from build123d import *

# Parameters (mm, degrees)
CHAMFER_1_SIZE      = 0.5
SKETCH_2_R          = 1.65
CUT_EXTRUDE_1_DEPTH = 10
SKETCH_3_R          = 1.65
CUT_EXTRUDE_2_DEPTH = 10


with BuildPart() as part:
    # 草图1 → 旋转1 (revolve)
    with BuildSketch(Plane(origin=(0, 0, 0), x_dir=(1, 0, 0), z_dir=(0, 1, 0))):
        Polygon((14, 8), (0, 8), (0, 2.5), (9, 2.5), (9, 4), (14, 4), align=None)
    revolve(axis=Axis((-5, 0, 0), (1, 0, 0)))

    # 倒角1
    chamfer_1_edges = [part.edges().sort_by_distance(p)[0] for p in [
        (14, 0, 4),
        (9, 0, 2.5),
        (0, 0, 2.5),
        (0, 0, 8),
        (14, 0, 8),
    ]]
    chamfer(chamfer_1_edges, length=CHAMFER_1_SIZE)

    # 草图2 → 切除-拉伸1 (cut)
    with BuildSketch(Plane(origin=(0, 0, 0), x_dir=(1, 0, 0), z_dir=(0, 1, 0))):
        with Locations((3, 0)):
            Circle(SKETCH_2_R)
        with Locations((11, 0)):
            Circle(SKETCH_2_R)
    extrude(amount=-CUT_EXTRUDE_1_DEPTH, mode=Mode.SUBTRACT)

    # 草图3 → 切除-拉伸2 (cut)
    with BuildSketch(Plane.XY):
        with Locations((3, 0)):
            Circle(SKETCH_3_R)
        with Locations((11, 0)):
            Circle(SKETCH_3_R)
    extrude(amount=-CUT_EXTRUDE_2_DEPTH, mode=Mode.SUBTRACT)


solid = part.part
Can you work these out from the model? Positions are in its coordinate system, mm. A direction names the side the tool comes from. Round coordinates to 2 decimals unless told otherwise and drop trailing zeros. Order: outer loops, then holes, each group sorted by start corner. A loop starts at its lowest first (then second) coordinate and runs counter-clockwise, first axis right, second up. Notation, with made-up numbers: M 60.5,62.25 L 110.5,62.25 A22 ccw 110.5,91.25 Z; hole C 2.5,15.5 d5. An arc over 180 degrees is marked long. Use a Markdown table: item, result.
1) I'm going to push flat-ended pins straight in: P1, Ø2.5, axis at y = 1, z = 0.5, coming from the +X side; P2, Ø3, axis at x = 11, y = -0.5, coming from the -Z side; P3, Ø6.5, axis at y = 0, z = 0, coming from the +X side; P4, Ø4, axis at x = 10, z = -2.5, coming from the +Y side. Where does each tip first touch, or does it pass through?
Geometry says:
| item | result |
|---|---|
| P1 | passes through |
| P2 | stops at z = -7.97 |
| P3 | stops at x = 9 |
| P4 | stops at y = 7.98 |
2) Imagine slicing it at C-C (x = 3). List the corners of the cut face in (y, z) for me, then the cut area to 3 significant figures.
Geometry says:
| item | result |
|---|---|
| outline | M -7.83,-1.65 A8 ccw -1.65,-7.83 L -1.65,-1.88 A2.5 cw -1.88,-1.65 Z; M -7.83,1.65 L -1.88,1.65 A2.5 cw long 1.65,-1.88 L 1.65,-7.83 A8 ccw long Z |
| area | 144 mm² |
3) If I drill on line 1 along X through (y, z) = (0, -6.65); line 2 along Y through (x, z) = (6.5, 0); line 3 along Y through (x, z) = (12, -4.5), over which ranges is the centre line in solid material (lowest first)?
Geometry says:
| item | result |
|---|---|
| line 1 | x = 0 to 1.35, 4.65 to 9.35, 12.65 to 14 |
| line 2 | y = -8 to -2.5, 2.5 to 8 |
| line 3 | y = -6.61 to -1.31, 1.31 to 6.61 |
4) Imagine slicing it at A-A (y = 0). Give the number of separate pieces and of enclosed holes in the cut face, then the cut area to 3 significant figures.
Geometry says:
| item | result |
|---|---|
| separate pieces | 4 |
| enclosed holes | 0 |
| area | 106 mm² |
5) If we mould it in two halves opening along Z, with no side actions, what happens to faces 1 (the face through (14, -5, 0)), 2 (the face through (6.91, -7.81, 1.73)), 3 (the face through (10.785, -5.794, -1.636))? For each: +Z half, -Z half, draft (parallel to the pull), parting line (faces both ways), or undercut.
Geometry says:
| item | result |
|---|---|
| face 1 | draft |
| face 2 | parting line |
| face 3 | undercut |
6) On a 3-axis mill with a long thin cutter (end or side, diameter ignored), from which of +Z, -Z, +X, -X, +Y, -Y can I reach the whole of each face in a straight line? I mean faces 4 (the face through (4.524, -4.898, 0.632)), 5 (the face through (4.524, -0.632, -4.896)), 6 (the face through (11.28, 2.7, 2.95)), 7 (the face through (0, -3.2, 0.1)), 8 (the face through (4.56, 1.69, 1.84)). Say none if no direction works.
Geometry says:
| item | result |
|---|---|
| face 4 | -Y |
| face 5 | -Z |
| face 6 | +X |
| face 7 | +Z, -Z, -X, +Y, -Y |
| face 8 | +X, -X |
7) Imagine slicing it at D-D (x = 8.75). List the corners of the cut face in (y, z) for me.
Geometry says:
| item | result |
|---|---|
| outline | C 0,0 d16; hole C 0,0 d5.5 |
